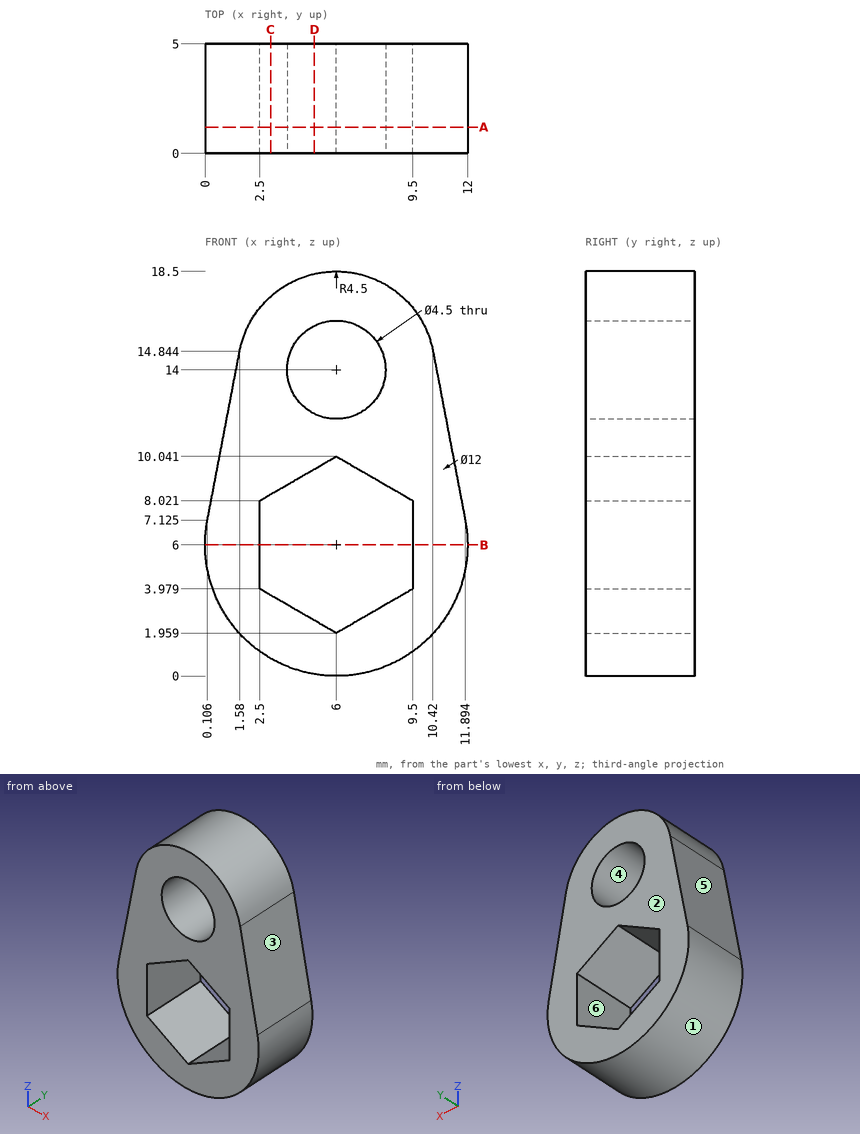
Study the drawing (mm; zero at the part's minimum x, y, z) and answer. A direction names the side the tool comes from. Round coordinates to 2 decimals unless told otherwise and drop trailing zeros. Write each loop counter-clockwise with the first axis right and the second up, starting at its lowest first coordinate (ties: lowest second). Pieces come first, ordered by that corner, then holes. Notation, with made-up numbers: (29, -30.5) -> (51, -30.5) arc R23 ccw to (51, 5.5) -> close; hole circle Ø10 at (89, 60). An arc over 180 degrees is marked (long way). Write each question's results on one line, items separated by ' | '.
Item 1: A cutting plane is placed at B-B, the plane z = 6. Determine the outline of the cut face in (x, y), plus the area to 3 significant figures.
Result set:
outline: (0, 0) -> (2.5, 0) -> (2.5, 5) -> (0, 5) -> close; (9.5, 0) -> (12, 0) -> (12, 5) -> (9.5, 5) -> close | area: 25.0 mm^2
Item 2: A cutting plane is placed at A-A, the plane y = 1.2. Count the separate pieces of the cut face and the enclosed holes in it.
Result set:
separate pieces: 1 | enclosed holes: 2
Item 3: Flat-ended cylindrical pins translate along their axes: P1, Ø1.5, axis at y = 3.5, z = 9.5, coming from the +X side; P2, Ø5, axis at x = 11, z = 13, coming from the -Y side; P3, Ø1, axis at y = 3.5, z = 2, coming from the +X side; P4, Ø2, axis at y = 1, z = 15.5, coming from the -X side. Find the tip coordinate at first contact, or state that the pin passes through.
Result set:
P1: x = 11.58 | P2: y = 0 | P3: x = 10.87 | P4: x = 1.51
Item 4: Which of the six approach directions +Z, -Z, +X, -X, +Y, -Y give full straight-line access (tool end or side, diameter ignored) to the marked faces 5 and 6?
Result set:
face 5: +Z, -X, +Y, -Y | face 6: +Y, -Y
Item 5: Find the intervals of material crossed by line 1 along X through (y, z) = (0.9, 6.25) (1 decimal); line 2 along Z through (x, y) = (5.5, 4.5) (1 decimal); line 3 along Z through (x, y) = (7.25, 2.3) (1 decimal), in increasing order. Write a range as [from, to].
Result set:
line 1: [0, 2.5], [9.5, 12] | line 2: [0, 2.2], [9.8, 11.8], [16.2, 18.5] | line 3: [0.1, 2.7], [9.3, 12.1], [15.9, 18.3]
Item 6: A cutting plane is placed at C-C, the plane x = 3. Determine the outline of the cut face in (y, z) (1 decimal).
Result set:
outline: (0, 0.8) -> (5, 0.8) -> (5, 3.7) -> (0, 3.7) -> close; (0, 8.3) -> (5, 8.3) -> (5, 17.4) -> (0, 17.4) -> close
Item 7: The mould has two halves that part along X. Classify the marked faces 1, 2, 3 and 4: +X half, -X half, draft (parallel to the pull), parting line (faces both ways), or undercut.
Result set:
face 1: parting line | face 2: draft | face 3: +X half | face 4: undercut
Item 8: A cutting plane is placed at D-D, the plane x = 5. Determine the outline of the cut face in (y, z) (1 decimal).
Result set:
outline: (0, 0.1) -> (5, 0.1) -> (5, 2.5) -> (0, 2.5) -> close; (0, 9.5) -> (5, 9.5) -> (5, 12) -> (0, 12) -> close; (0, 16) -> (5, 16) -> (5, 18.4) -> (0, 18.4) -> close
